```python
from build123d import *

# Parameters (mm, degrees)
SHANK_TIP_CHAMFER_SIZE          = 0.3
COUNTERSUNK_HEAD_CHAMFER_SIZE   = 1.65
COUNTERSUNK_HEAD_CHAMFER_SIZE_2 = 1.55
HEX_DRIVE_CUT_DEPTH             = 1.023


with BuildPart() as part:
    # Screw Section → Screw Blank Revolve (revolve)
    with BuildSketch(Plane(origin=(0, 0, 0), x_dir=(1, 0, 0), z_dir=(0, 1, 0))):
        Polygon((0, 12), (1.2, 12), (1.2, 1.65), (2.75, 1.65), (2.75, 0), (0, 0), align=None)
    revolve(axis=Axis((0, 0, 10.123), (0, 0, -1)))

    # Shank Tip Chamfer
    shank_tip_chamfer_edges = [part.edges().sort_by_distance(p)[0] for p in [
        (-1.2, 0, -12),
    ]]
    chamfer(shank_tip_chamfer_edges, length=SHANK_TIP_CHAMFER_SIZE)

    # Countersunk Head Chamfer
    # the kernel refuses this chamfer: 1.65, 1.55 mm, written as the material it takes off along each edge
    with BuildSketch(Plane(origin=(0, 0, -1.65), x_dir=(1, 0, 0), z_dir=(0, 1, 0))) as countersunk_head_chamfer_piece_1_section:
        Polygon((2.75 - COUNTERSUNK_HEAD_CHAMFER_SIZE, 0), (2.75, -COUNTERSUNK_HEAD_CHAMFER_SIZE_2), (2.75, 0), align=None)
    countersunk_head_chamfer_piece_1 = revolve(axis=Axis((0, 0, -1.65), (0, 0, -1)), mode=Mode.PRIVATE)
    countersunk_head_chamfer_piece_1 = countersunk_head_chamfer_piece_1 - Plane(origin=(0, 0, -0.825037094), x_dir=(1, 0, 0), z_dir=(0, 0, 1)) * Cylinder(1.2, 11, mode=Mode.PRIVATE)
    add(countersunk_head_chamfer_piece_1, mode=Mode.SUBTRACT)

    # Hex Drive Sketch → Hex Drive Cut (cut)
    with BuildSketch(Plane.XY):
        Polygon((1.154700538, 0), (0.577350269, 1), (-0.577350269, 1), (-1.154700538, 0), (-0.577350269, -1), (0.577350269, -1), align=None)
    extrude(amount=-HEX_DRIVE_CUT_DEPTH, mode=Mode.SUBTRACT)


solid = part.part
```
Here's how the part is built. I have some questions about the finished solid (model axes, mm). A direction names the side the tool comes from. Round coordinates to 2 decimals unless told otherwise and drop trailing zeros. Write each loop counter-clockwise with the first axis right and the second up, starting at its lowest first coordinate (ties: lowest second). Pieces come first, ordered by that corner, then holes.
Q1. If we section it at B-B on z = -6.5: Write out the boundary of the cut face in (x, y).
Q2. Please list where these lines run through material, in increasing order: probe 1 along Z at (x, y) = (-0.75, -0.3); probe 2 along X at (y, z) = (-0.75, -0.75); probe 3 along X at (y, z) = (-0.05, -4.25).
Q3. If we mould it in two halves opening along X, with no side actions, what happens to faces 1 (the flat face through (0, -1, -0.5)), 2 (the flat face through (0, 0, -12))? For each: +X half, -X half, draft (parallel to the pull), parting line (faces both ways), or undercut.
Q4. Will these pins go through, and if not, where does the flat tip stop? P1, Ø3, axis at y = -1.5, z = -10.5, coming from the -X side; P2, Ø2, axis at x = -1.5, z = -4, coming from the +Y side.
Q5. If we section it at A-A on x = 0: Write out the boundary of the cut face in (y, z), plus the area to 3 significant figures.
Q6. Which directions (+Z, -Z, +X, -X, +Y, -Y) give clear straight access to the entire face, cutting with the end or side of a thin tool? Please do faces 3 (the flat face through (0, 1.2, 0)), 4 (the flat face through (0, 0, -1.023)).
Answer below:
1. outline: circle Ø2.4 at (0, 0)
2. probe 1: z = -12 to -1.02
2. probe 2: x = -1.92 to -0.72, 0.72 to 1.92
2. probe 3: x = -1.2 to 1.2
3. face 1: undercut
3. face 2: draft
4. P1: stops at x = -1.2
4. P2: stops at y = 1.09
5. outline: (-2.75, -0.1) - (-1.2, -1.56) - (-1.2, -11.7) - (-0.9, -12) - (0.9, -12) - (1.2, -11.7) - (1.2, -1.56) - (2.75, -0.1) - (2.75, 0) - (1, 0) - (1, -1.02) - (-1, -1.02) - (-1, 0) - (-2.75, 0) - close
5. area: 29.2 mm2
6. face 3: +Z, +X, -X, +Y, -Y
6. face 4: +Z
